Input: part model. Units: mm. Frame: model coordinates. A direction names the side the tool comes from. Give positions to 0.01 mm unless a question says otherwise; leave off trailing zeros. Write each loop counter-clockwise with the first axis right and the second up, starting at its lowest first coordinate (ties: lowest second). Pieces come first, ordered by that corner, then holes. Notation, with made-up numbers: M 19,85 L 68,85 A36 cw 68,121 Z; hole C -16.75,75.5 d8. An arc over 180 degrees is marked long. Use CSV: the item, a comma, the result in double quotes. Start each with the question number.
from build123d import *

# Parameters (mm, degrees)
SZKIC1_R                         = 1.4
DODANIE_WYCI_GNI_CIE1_DEPTH      = 54
DODANIE_WYCI_GNI_CIE1_DEPTH_BACK = 54
SZKIC2_R                         = 4
DODANIE_WYCI_GNI_CIE2_DEPTH      = 49
DODANIE_WYCI_GNI_CIE2_DEPTH_BACK = 49
SFAZOWANIE4_SIZE                 = 2.5


with BuildPart() as part:
    # Szkic1 → Dodanie-wyci_gni_cie1 (new body, two sides)
    with BuildSketch(Plane.XY) as dodanie_wyci_gni_cie1_sk:
        Circle(SZKIC1_R)
    extrude(amount=DODANIE_WYCI_GNI_CIE1_DEPTH)
    extrude(dodanie_wyci_gni_cie1_sk.sketch, amount=-DODANIE_WYCI_GNI_CIE1_DEPTH_BACK)

    # Szkic2 → Dodanie-wyci_gni_cie2 (add, two sides)
    with BuildSketch(Plane.XY) as dodanie_wyci_gni_cie2_sk:
        Circle(SZKIC2_R)
    extrude(amount=DODANIE_WYCI_GNI_CIE2_DEPTH)
    extrude(dodanie_wyci_gni_cie2_sk.sketch, amount=-DODANIE_WYCI_GNI_CIE2_DEPTH_BACK)

    # Sfazowanie4
    sfazowanie4_edges = [part.edges().sort_by_distance(p)[0] for p in [
        (-4, 0, -49),
        (-4, 0, 49),
    ]]
    chamfer(sfazowanie4_edges, length=SFAZOWANIE4_SIZE)


solid = part.part
Q1. Set-up query: faces 1 (the flat face through (0, 0, -54)), 2 (the cylindrical face through (-1.4, 0.06, 51.54)), 3 (the cylindrical face through (-1.4, 0.06, -51.46)). Return all of +Z, -Z, +X, -X, +Y, -Y with unobstructed straight access to the full face (end or side cutting, diameter ignored); none if empty.
Q2. Section C-C, the plane z = -11.5. Return the cut outline in (x, y).
Q3. Section A-A, the plane y = 0. Return the cut outline in (x, z).
Q4. First-contact query: pin 1 Ø2 at (x, y) = (-0.5, -3) entering from -Z; pin 2 Ø1.5 at (y, z) = (-1, 9.5) entering from -X; pin 3 Ø1 at (x, z) = (1, 37.5) entering from -Y. Flat tips, straight axial feed; report the tip coordinate or a pass-through.
Q5. Material intervals for L1, parallel to X at y = 0.25, z = -16.5; L2, parallel to Y at x = 3.5, z = -38; L3, parallel to Y at x = 1.25, z = -36, sorted ascending. Write a range as [from, to].
Check result:
1,face 1,"-Z, +X, -X, +Y, -Y"
1,face 2,"+Z"
1,face 3,"-Z"
2,outline,"C 0,0 d8"
3,outline,"M -4,-46.5 L -1.5,-49 L -1.4,-49 L -1.4,-54 L 1.4,-54 L 1.4,-49 L 1.5,-49 L 4,-46.5 L 4,46.5 L 1.5,49 L 1.4,49 L 1.4,54 L -1.4,54 L -1.4,49 L -1.5,49 L -4,46.5 Z"
4,pin 1,"stops at z = -48.46"
4,pin 2,"stops at x = -3.99"
4,pin 3,"stops at y = -3.97"
5,L1,"x = [-3.99, 3.99]"
5,L2,"y = [-1.94, 1.94]"
5,L3,"y = [-3.8, 3.8]"
